from build123d import *

# Parameters (mm, degrees)
F0_R     = 82.200054
F0_R_2   = 75.168318
F1_DEPTH = 25.4
F2_R     = 7.62
F3_DEPTH = 7.62


with BuildPart() as f1:
    # F0 (on Top) → F1 (new body)
    with BuildSketch(Plane.XY):
        Circle(F0_R)
        Circle(F0_R_2, mode=Mode.SUBTRACT)
        Circle(F0_R_2)
        with BuildLine():
            ThreePointArc((37.00019, -57.652773), (-54.364996, 2.604364), (41.772287, 54.912514))
            ThreePointArc((41.772287, 54.912514), (-13.536125, 0.873463), (37.00019, -57.652773))
        make_face(mode=Mode.SUBTRACT)
    extrude(amount=F1_DEPTH)

    # F2
    f2_edges = [f1.edges().sort_by_distance(p)[0] for p in [
        (-82.200054, 0, 25.4),
        (-82.200054, 0, 0),
    ]]
    fillet(f2_edges, radius=F2_R)

    # F0 (on Top) → F3 (join)
    with BuildSketch(Plane.XY):
        with BuildLine():
            ThreePointArc((37.00019, -57.652773), (-13.536125, 0.873463), (41.772287, 54.912514))
            ThreePointArc((41.772287, 54.912514), (-54.364996, 2.604364), (37.00019, -57.652773))
        make_face()
    extrude(amount=F3_DEPTH)


solid = f1.part
The model under review builds one solid part; all positions refer to its coordinate system, in mm. Give positions to 0.01 mm unless a question says otherwise; leave off trailing zeros. Order: outer loops, then holes, each group sorted by start corner. A loop starts at its lowest first (then second) coordinate and runs counter-clockwise, first axis right, second up. Notation, with made-up numbers: M -8,4.5 L 46,4.5 A18 ccw 46,15.5 Z; hole C 17,-22 d10. An arc over 180 degrees is marked long. Use one line per item in the form item = value. Start each with the question number.
Item 1: The part is to be moulded in two halves that separate along Y. For faces 1 (the cylindrical face through (-54.416, 0.764, 16.386)), 2 (the flat face through (-1, 1, 0)), 3 (the flat face through (-18, 1, 7.62)), 4 (the cylindrical face through (-10.7, 81.5, 12.6)), say which applies: pulls with the +Y half, pulls with the -Y half, needs draft (parallel to the pull), parting line crosses it, or undercut.
Item 2: Insertion check: pin 1 Ø3 at (y, z) = (-45.5, 6) entering from -X; pin 2 Ø1 at (x, y) = (-34, -30.5) entering from +Z; pin 3 Ø2 at (y, z) = (59.5, 4) entering from -X; pin 4 Ø1.5 at (x, y) = (-42.5, 42.5) entering from -Z. Each pin has a flat end and moves straight along its axis. Give the tip position at first contact, or say it passes through.
Item 3: To check wall thickness, follow line 1 along Y through (x, z) = (20, 21); line 2 along Y through (x, z) = (28, 22.25); line 3 along Z through (x, y) = (-3.5, 50). State the ranges of each line that lie inside material, in increasing order. Write a range as from..to.
Item 4: We need section A-A on x = 0. Give the boundary of the cut face in (y, z), plus the area to 3 significant figures.
Item 5: We need section C-C on z = 3.5. Give the boundary of the cut face in (x, y), plus the area to 3 significant figures.
Item 6: We need section B-B on y = 0. Give the boundary of the cut face in (x, z), plus the area to 3 significant figures.
Completed:
q1.face_1 = undercut
q1.face_2 = needs draft
q1.face_3 = undercut
q1.face_4 = parting line crosses it
q2.pin_1 = -69.28
q2.pin_2 = 7.62
q2.pin_3 = -56.65
q2.pin_4 = 0
q3.line_1 = -78.99..-63.04, -53.12..50.09, 62.84..78.99
q3.line_2 = -75.74..-61.16, -55.97..52.93, 60.96..75.74
q3.line_3 = 0..7.62
q4.outline = M -82.2,7.62 A7.62 ccw -74.58,0 L 74.58,0 A7.62 ccw 82.2,7.62 L 82.2,17.78 A7.62 ccw 74.58,25.4 L 63.03,25.4 L 63.03,7.62 L 35.21,7.62 L 35.21,25.4 L -38.25,25.4 L -38.25,7.62 L -63.23,7.62 L -63.23,25.4 L -74.58,25.4 A7.62 ccw -82.2,17.78 Z
q4.area = 3,190 mm²
q5.outline = C 0,0 d161.98
q5.area = 20,600 mm²
q6.outline = M -82.2,7.62 A7.62 ccw -74.58,0 L 74.58,0 A7.62 ccw 82.2,7.62 L 82.2,17.78 A7.62 ccw 74.58,25.4 L -13.57,25.4 L -13.57,7.62 L -54.42,7.62 L -54.42,25.4 L -74.58,25.4 A7.62 ccw -82.2,17.78 Z
q6.area = 3,400 mm²
